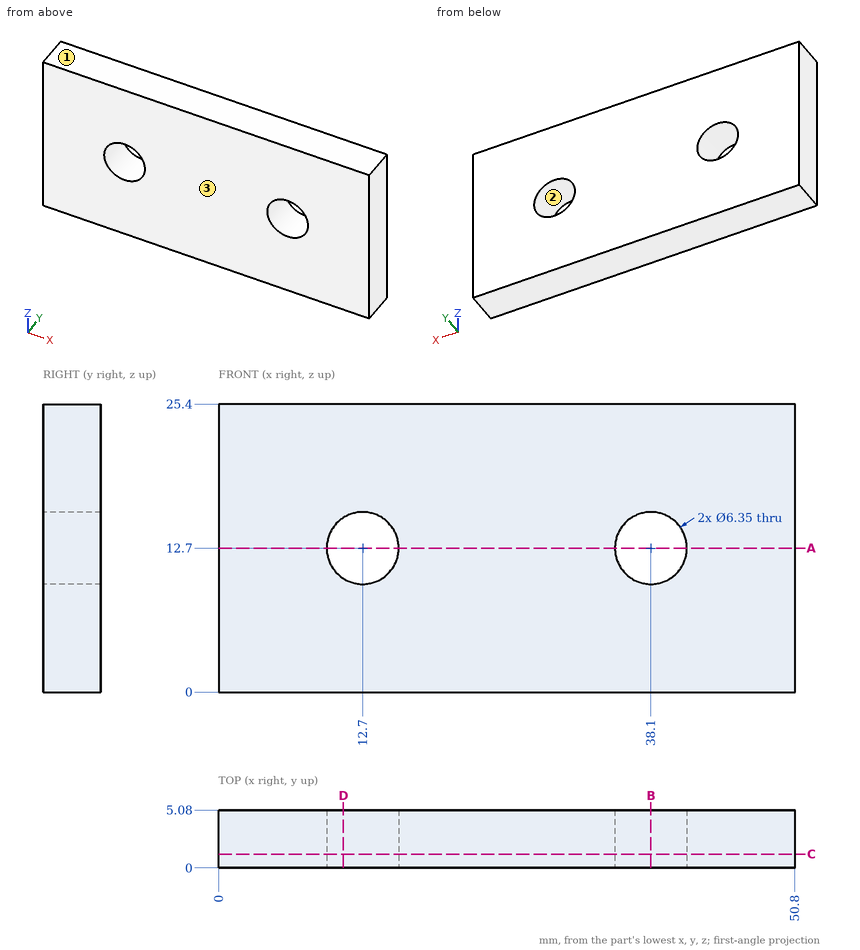
Geometry check sheet. Reference: drawing and pictorial views, mm from the part's lowest x, y, z. Coordinates: 2 decimals unless noted, no trailing zeros. Order: outer loops, then holes, each group sorted by start corner. A loop starts at its lowest first (then second) coordinate and runs counter-clockwise, first axis right, second up.
1. Sectioned sample at C-C, the plane y = 1.2. Record the cut outline in (x, z) (3 decimals).
Results found:
outline: (0, 0) - (50.8, 0) - (50.8, 25.4) - (0, 25.4) - close; hole circle Ø6.35 at (12.7, 12.7); hole circle Ø6.35 at (38.1, 12.7)
2. Sectioned sample at B-B, the plane x = 38.1. Record the cut outline in (y, z) (3 decimals), and give its area (3 significant figures).
Results found:
outline: (0, 0) - (5.08, 0) - (5.08, 9.525) - (0, 9.525) - close; (0, 15.875) - (5.08, 15.875) - (5.08, 25.4) - (0, 25.4) - close
area: 96.8 mm2
3. Scan lines: line 1 (X direction, y = 3.2, z = 12.7) (3 decimals); line 2 (Z direction, x = 12.7, y = 2.8) (3 decimals); line 3 (X direction, y = 3.6, z = 15.25). Record each from-to range of solid material in increasing order.
Results found:
line 1: x = 0 to 9.525, 15.875 to 34.925, 41.275 to 50.8
line 2: z = 0 to 9.525, 15.875 to 25.4
line 3: x = 0 to 10.81, 14.59 to 36.21, 39.99 to 50.8
4. Release check for a two-part mould opening along Z. For the marked faces 1, 2 and 3 record: +Z half, -Z half, draft (parallel to the pull), parting line (faces both ways), or undercut.
Results found:
face 1: +Z half
face 2: undercut
face 3: draft
5. Sectioned sample at D-D, the plane x = 11. Record the cut outline in (y, z).
Results found:
outline: (0, 0) - (5.08, 0) - (5.08, 10.02) - (0, 10.02) - close; (0, 15.38) - (5.08, 15.38) - (5.08, 25.4) - (0, 25.4) - close
6. Sectioned sample at A-A, the plane z = 12.7. Record the cut outline in (x, y) (3 decimals), and give its area (3 significant figures).
Results found:
outline: (0, 0) - (9.525, 0) - (9.525, 5.08) - (0, 5.08) - close; (15.875, 0) - (34.925, 0) - (34.925, 5.08) - (15.875, 5.08) - close; (41.275, 0) - (50.8, 0) - (50.8, 5.08) - (41.275, 5.08) - close
area: 194 mm2
